from build123d import *

# Parameters (mm, degrees)
CROQUIS1_R              = 1.5
CROQUIS1_R_2            = 11.9
SALIENTE_EXTRUIR1_DEPTH = 5.5


with BuildPart() as part:
    # Croquis1 → Saliente-Extruir1 (new body)
    with BuildSketch(Plane.XY):
        with BuildLine():
            Line((-20, 20), (20, 20))
            ThreePointArc((20, 20), (23.535533906, 18.535533906), (25, 15))
            Line((25, 15), (25, -15))
            ThreePointArc((25, -15), (23.535533906, -18.535533906), (20, -20))
            Line((20, -20), (-20, -20))
            ThreePointArc((-20, -20), (-23.535533906, -18.535533906), (-25, -15))
            Line((-25, -15), (-25, 15))
            ThreePointArc((-25, 15), (-23.535533906, 18.535533906), (-20, 20))
        make_face()
        with Locations((-20, 15)):
            Circle(CROQUIS1_R, mode=Mode.SUBTRACT)
        Circle(CROQUIS1_R_2, mode=Mode.SUBTRACT)
        with Locations((-20, -15)):
            Circle(CROQUIS1_R, mode=Mode.SUBTRACT)
        with Locations((20, -15)):
            Circle(CROQUIS1_R, mode=Mode.SUBTRACT)
        with Locations((20, 15)):
            Circle(CROQUIS1_R, mode=Mode.SUBTRACT)
    extrude(amount=SALIENTE_EXTRUIR1_DEPTH)


solid = part.part
Part model, mm, in its own coordinate system. Give positions to 0.01 mm unless a question says otherwise; leave off trailing zeros. Loops run counter-clockwise (first coordinate to the right, second up) from the corner with the lowest first, then second, coordinate; pieces in that order, holes last.
(1) Pull direction Y, two halves, no side cores. Call faces 1 (the flat face through (11.5, -4.2, 0)), 2 (the cylindrical face through (-21.5, -14.93, 2.71)), 3 (the flat face through (0, -20, 3)): pulls with the +Y half, pulls with the -Y half, needs draft (parallel to the pull), parting line crosses it, or undercut.
Return value:
face 1: needs draft
face 2: undercut
face 3: pulls with the -Y half
(2) Band-saw the part on C-C (x = 0). Write the cut outline in (y, z).
Return value:
outline: (-20, 0) - (-11.9, 0) - (-11.9, 5.5) - (-20, 5.5) - close; (11.9, 0) - (20, 0) - (20, 5.5) - (11.9, 5.5) - close
(3) Pin check, flat tip, straight feed: pin 1 (5 mm diameter, centred on x = -20, y = 15, fed in from +Z). Stop position of the tip, or through.
Return value:
pin 1: stops at z = 5.5
(4) Band-saw the part on B-B (z = 1.4). Write the cut outline in (x, y), and give its area (3 significant figures).
Return value:
outline: (-25, -15) arc R5 ccw to (-20, -20) - (20, -20) arc R5 ccw to (25, -15) - (25, 15) arc R5 ccw to (20, 20) - (-20, 20) arc R5 ccw to (-25, 15) - close; hole circle Ø3 at (-20, -15); hole circle Ø3 at (-20, 15); hole circle Ø23.8 at (0, 0); hole circle Ø3 at (20, -15); hole circle Ø3 at (20, 15)
area: 1,510 mm2
(5) Band-saw the part on A-A (y = 0). Write the cut outline in (x, z), and give its area (3 significant figures).
Return value:
outline: (-25, 0) - (-11.9, 0) - (-11.9, 5.5) - (-25, 5.5) - close; (11.9, 0) - (25, 0) - (25, 5.5) - (11.9, 5.5) - close
area: 144 mm2
(6) Drill centre lines: line 1 along Y through (x, z) = (21, 2.1); line 2 along Y through (x, z) = (0, 3.7); line 3 along X through (y, z) = (9, 4.6). Where is each one in solid material? Low to high.
Return value:
line 1: y = -19.9 to -16.12, -13.88 to 13.88, 16.12 to 19.9
line 2: y = -20 to -11.9, 11.9 to 20
line 3: x = -25 to -7.79, 7.79 to 25
